from build123d import *

# Parameters (mm, degrees)
F0_W     = 19.05
F0_H     = 19.05
F1_DEPTH = 19.05
F2_DEPTH = 19.05
F4_DEPTH = 19.05
F3_W     = 19.05
F3_H     = 19.05
F5_DEPTH = 19.05
F6_DEPTH = 19.05
F7_W     = 19.05
F7_H     = 19.05
F8_DEPTH = 19.05


with BuildPart() as f1:
    # F0 (on Top) → F1 (new body)
    with BuildSketch(Plane.XY):
        with Locations((9.525, 9.525)):
            Rectangle(F0_W, F0_H)
    extrude(amount=F1_DEPTH)

    # F2 (add): a face of the model
    f2_faces = [f1.faces().sort_by_distance(p)[0] for p in [
        (9.525, 19.05, 9.525),
    ]]
    extrude(f2_faces, amount=F2_DEPTH)

    # F4 (add): a face of the model
    f4_faces = [f1.faces().sort_by_distance(p)[0] for p in [
        (9.525, 38.1, 9.525),
    ]]
    extrude(f4_faces, amount=F4_DEPTH)

    # F3 (on face) → F5 (join)
    with BuildSketch(Plane.XY.offset(19.05)):
        with Locations((9.525, 9.525)):
            Rectangle(F3_W, F3_H)
    extrude(amount=F5_DEPTH)

    # F6 (add): a face of the model
    f6_faces = [f1.faces().sort_by_distance(p)[0] for p in [
        (9.525, 9.525, 38.1),
    ]]
    extrude(f6_faces, amount=F6_DEPTH)

    # F7 (on face) → F8 (join)
    with BuildSketch(Plane(origin=(0, 19.05, 0), x_dir=(-1, 0, 0), z_dir=(0, 1, 0))):
        with Locations((-9.525, 28.575)):
            Rectangle(F7_W, F7_H)
    extrude(amount=F8_DEPTH)


solid = f1.part
The model under review builds one solid part; all positions refer to its coordinate system, in mm. A direction names the side the tool comes from. Round coordinates to 2 decimals unless told otherwise and drop trailing zeros. Loops run counter-clockwise (first coordinate to the right, second up) from the corner with the lowest first, then second, coordinate; pieces in that order, holes last. Notation, with made-up numbers: (1, -10) -> (5, -10) arc R23 ccw to (5, 14) -> close; hole circle Ø4 at (-9.75, 26.25). An arc over 180 degrees is marked (long way). One line per question, with ' | ' between items. Start each with the question number.
Item 1: Add section B-B, the plane y = 45.5. Write out the cut boundary in (x, z).
Item 2: For pin 1 (5.5 mm diameter, centred on x = 9, y = 47.5, fed in from +Z); pin 2 (9.5 mm diameter, centred on x = 11.5, z = 49, fed in from +Y); pin 3 (8 mm diameter, centred on x = 3.5, z = 40.5, fed in from +Y), all flat-tipped, find the tip position at first contact; note any pin that passes through.
Item 3: Wall thickness on line 1 along Z through (x, y) = (7, 30); line 2 along Z through (x, y) = (5, 43): over which ranges is each line inside the solid? List them lowest first. Write a range as [from, to].
Item 4: Machinability: for faces 1 (the face through (9, 47, 19.05)), 2 (the face through (0, 22, 22)), which of the approach directions +Z, -Z, +X, -X, +Y, -Y give a long, thin tool a straight path to every point of the face, cutting with its end or side? Answer none if there is none.
Item 5: Add section A-A, the plane x = 14. Write out the cut boundary in (y, z), then the cut area to 3 significant figures.
Return value:
1) outline: (0, 0) -> (19.05, 0) -> (19.05, 19.05) -> (0, 19.05) -> close
2) pin 1: stops at z = 19.05 | pin 2: stops at y = 19.05 | pin 3: stops at y = 38.1
3) line 1: z = [0, 38.1] | line 2: z = [0, 19.05]
4) face 1: +Z, +X, -X, +Y | face 2: +Z, -Z, -X, +Y, -Y
5) outline: (0, 0) -> (57.15, 0) -> (57.15, 19.05) -> (38.1, 19.05) -> (38.1, 38.1) -> (19.05, 38.1) -> (19.05, 57.15) -> (0, 57.15) -> close | area: 2,180 mm2
